from build123d import *

# Parameters (mm, degrees)
F0_W     = 2.54
F0_H     = 12.7
F1_ANGLE = 180
F3_DEPTH = 6.35
F4_R     = 1.27


with BuildPart() as f1:
    # F0 (on Front) → F1 (revolve)
    with BuildSketch(Plane.XZ):
        with BuildLine():
            Line((-17.4625, -13.97), (-17.4625, 13.97))
            ThreePointArc((-17.4625, 13.97), (-18.392436, 16.215064), (-20.6375, 17.145))
            Line((-20.6375, 17.145), (-23.8125, 17.145))
            Line((-23.8125, 17.145), (-23.8125, 13.97))
            ThreePointArc((-23.8125, 13.97), (-23.440526, 13.071974), (-22.5425, 12.7))
            Line((-22.5425, 12.7), (-22.5425, -12.7))
            ThreePointArc((-22.5425, -12.7), (-23.440526, -13.071974), (-23.8125, -13.97))
            Line((-23.8125, -13.97), (-23.8125, -17.145))
            Line((-23.8125, -17.145), (-20.6375, -17.145))
            ThreePointArc((-20.6375, -17.145), (-18.392436, -16.215064), (-17.4625, -13.97))
        make_face()
        with Locations((-20.0025, 0)):
            Rectangle(F0_W, F0_H, mode=Mode.SUBTRACT)
    revolve(axis=Axis((0, 0, 0), (0, 0, -1)), revolution_arc=F1_ANGLE)

    # F2 (on Top) → F3 (join, symmetric)
    with BuildSketch(Plane.XY):
        with BuildLine():
            Line((-18.104011, 4.811585), (-20.721195, 4.811585))
            ThreePointArc((-20.721195, 4.811585), (-21.134224, 2.421533), (-21.2725, 0))
            ThreePointArc((-21.2725, 0), (-21.047769, -1.867615), (-20.386407, -3.628606))
            Line((-20.386407, -3.628606), (-18.7325, -3.628606))
            Line((-18.7325, -3.628606), (-18.7325, 0))
            ThreePointArc((-18.7325, 0), (-18.574713, 2.426229), (-18.104011, 4.811585))
        make_face()
    extrude(amount=F3_DEPTH, both=True)

    # F4
    f4_edges = [f1.edges().sort_by_distance(p)[0] for p in [
        (0, 22.5425, 12.7),
        (0, 22.5425, -12.7),
        (0, 23.8125, 17.145),
        (0, 23.8125, -17.145),
    ]]
    fillet(f4_edges, radius=F4_R)


solid = f1.part
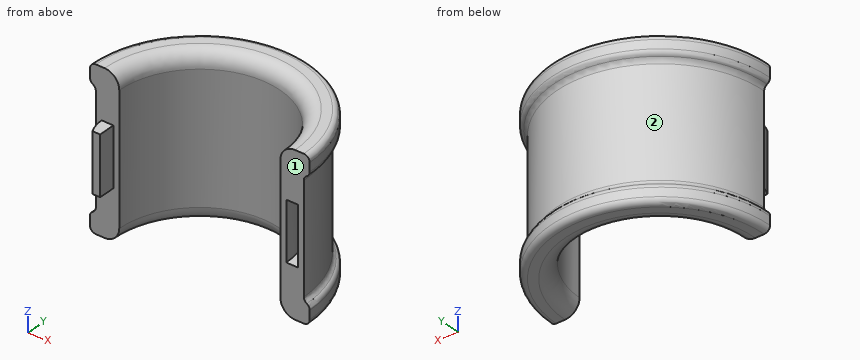
Model file for the job. Use its own axes, mm. Face numbers are marked on the shaded views. Give positions to 0.01 mm unless a question says otherwise; leave off trailing zeros. Write each loop counter-clockwise with the first axis right and the second up, starting at its lowest first coordinate (ties: lowest second). Pieces come first, ordered by that corner, then holes. Notation, with made-up numbers: (-30.5, 81) - (10.5, 81) arc R21 ccw to (10.5, 103) - close; hole circle Ø3 at (3.5, 22.5). An arc over 180 degrees is marked (long way). Answer as CSV lines item,"result".
1. Band-saw the part on D-D (z = -11). Write the cut outline in (x, y) (1 decimal), and give its area (3 significant figures).
Responses:
outline,"(-22.5, 0) - (-17.5, 0) arc R17.5 cw to (17.5, 0) - (22.5, 0) arc R22.5 ccw to start"
area,"319 mm2"
2. Two-plate mould, pull along Z, no slides. Class the marked faces 1 and 2: +Z half, -Z half, draft (parallel to the pull), parting line (faces both ways), or undercut.
Responses:
face 1,"draft"
face 2,"undercut"
3. Drill centre lines: L1, parallel to Y at x = 0, z = -1.5; L2, parallel to X at y = 8.25, z = -10; L3, parallel to X at y = 4, z = 15. Where is each one in solid material? Low to high. Write a range as [from, to].
Responses:
L1,"y = [17.46, 18.73], [21.27, 22.54]"
L2,"x = [-20.98, -15.39], [15.39, 20.98]"
L3,"x = [-23.47, -17.17], [17.17, 23.47]"
4. Band-saw the part on B-B (y = 15.75). Count the separate pieces of the cut face and the enclosed holes in it, and give its area (3 significant figures).
Responses:
separate pieces,"2"
enclosed holes,"2"
area,"493 mm2"
5. Pin check, flat tips, straight feed: pin 1 (3 mm diameter, centred on y = 6, z = -4.5, fed in from -X); pin 2 (2 mm diameter, centred on y = 20, z = 2.5, fed in from +X); pin 3 (12 mm diameter, centred on y = -0.5, z = 6.5, fed in from +X); pin 4 (5 mm diameter, centred on x = -21.5, z = 1, fed in from -Y). Stop position of each tip, or through.
Responses:
pin 1,"stops at x = -22.09"
pin 2,"stops at x = 12.13"
pin 3,"stops at x = 22.76"
pin 4,"stops at y = -3.63"
6. Band-saw the part on A-A (z = -4.5). Write the cut outline in (x, y) (1 decimal), and give its area (3 significant figures).
Responses:
outline,"(-22.5, 0) - (-21.3, 0) arc R7.9 ccw to (-20.4, -3.6) - (-18.7, -3.6) - (-18.7, 0) - (-17.5, 0) arc R17.5 cw to (17.5, 0) - (18.7, 0) arc R18.7 ccw to (-18.1, 4.8) - (-20.7, 4.8) arc R21.3 cw to (21.3, 0) - (22.5, 0) arc R22.5 ccw to start"
area,"180 mm2"
